For this review, take the finished solid that the model builds, in its own axes (mm). Face numbers are marked on the shaded views. A direction names the side the tool comes from. Coordinates: 2 decimals unless noted, no trailing zeros. Write each loop counter-clockwise with the first axis right and the second up, starting at its lowest first coordinate (ties: lowest second). Pieces come first, ordered by that corner, then holes. Notation, with made-up numbers: M 49.25,17.25 L 54.25,17.25 A25 cw 54.25,33.25 Z; hole C 53,-0.75 d9. An arc over 180 degrees is marked long. One line per question, with ' | ' between items.
Autodesk Inventor part; units mm, degrees
ref_plane "YZ Plane" through (0, 0, 0) normal (1, 0, 0) x (0, 1, 0)
ref_plane "XZ Plane" through (0, 0, 0) normal (0, 1, 0) x (-1, 0, 0)
ref_plane "XY Plane" through (0, 0, 0) normal (0, 0, 1) x (1, 0, 0)
sketch "Sketch1" plane through (0, 0, 0) normal (0, 0, 1) x (1, 0, 0)
  line L0 (-33.6, 0) -> (33.6, 0) construction
  line L1 (0, -33.6) -> (0, 33.6) construction
  circle A0 centre (0, 0) radius 24
  dimension "d0" = 48
extrude "Выдавливание1" add sketch "Sketch1" along normal blind 10
hole "Отверстие1" at (0, 0, 10) direction (0, 0, -1) diameter 28.376 end through all
sketch "Sketch2" plane through (0, 0, 10) normal (0, 0, 1) x (1, 0, 0)
  circle A0 centre (0, 0) radius 24
  circle A1 centre (0, 0) radius 19 construction
  line L0 (-33.6, 0) -> (33.6, 0) construction
  line L1 (0, -33.6) -> (0, 33.6) construction
  point P0 (-19, 0)
  point P1 (0, 19)
  point P2 (19, 0)
  point P3 (0, -19)
  dimension "d13" = 38
hole "Отверстие2" at (-19, 0, 10) at (0, 19, 10) at (19, 0, 10) at (0, -19, 10) direction (0, 0, -1) diameter 4.5 depth 7 tip angle 118
chamfer "Фаска1" distance 0.6 angle 45 4 edges at (0, -16.75, 10) (-19, 2.25, 10) (19, 2.25, 10) (0, 21.25, 10)
chamfer "Фаска2" distance 1 angle 45 2 edges at (-24, 0, 10) (-24, 0, 0)
sketch "Sketch3" plane through (0, 0, 0) normal (1, 0, 0) x (0, 1, 0)
  line L0 (-14.188, 0) -> (-14.188, 10) construction
  line L1 (14.188, 0) -> (14.188, 10) construction
  line L2 (-15, 10) -> (0, -5)
  line L3 (-15, 10) -> (0, 10)
  line L4 (0, 10) -> (0, -5)
  line L5 (0, -9) -> (0, 19) construction
  line L6 (-15.6074, 5) -> (15.0846, 5) construction
  line L7 (-21.7458, 0) -> (21.223, 0) construction
  line L8 (-15, 0) -> (0, 15)
  line L9 (-15, 0) -> (0, 0)
  line L10 (0, 0) -> (0, 15)
  point P0 (14.188, 5)
  dimension "d30" = 10
  dimension "d31" = 30
  dimension "d32" = 45
  dimension "d34" = 5
revolve "Вращение1" cut sketch "Sketch3" angle 360 about axis through (0, 0, -10) along (0, 0, 1)
equation "\"d0\" = D_L"
equation "\"d2\" = m_"
equation "\"d13\" = D_x"
equation "\"d14\" = d1"
equation "\"d16\" = d1"
equation "\"d19\" = h_"
equation "\"d21\" = c1"
equation "\"d24\" = c_"
equation "\"d30\" = m_"
equation "\"d31\" = d_"
equation "\"d34\" = 0.5 * m_"
equation "\"d_\" = 30"
equation "\"D_L\" = 48"
equation "\"D_x\" = 38"
equation "\"d1\" = 4.5"
equation "\"m_\" = 10"
equation "\"h_\" = 7"
equation "\"c_\" = 1"
equation "\"c1\" = 0.6"
properties part number "Гайка M30x1.5 6H ГОСТ 6393-73" material "Сталь, мягкая"
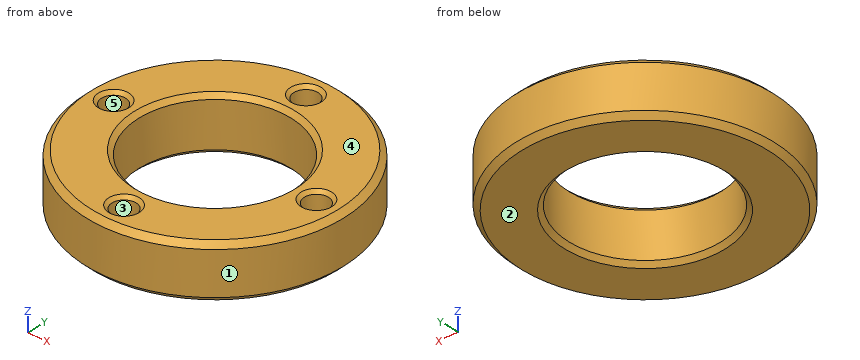
1) Machinability: for the marked faces 4 and 5, which of the approach directions +Z, -Z, +X, -X, +Y, -Y give a long, thin tool a straight path to every point of the face, cutting with its end or side? Answer none if there is none.
Responses:
face 4: +Z, +X, -X, +Y, -Y | face 5: +Z
2) Insertion check: pin 1 Ø4 at (x, y) = (0, -19) entering from -Z; pin 2 Ø3.5 at (x, y) = (0, 19) entering from +Z; pin 3 Ø5 at (x, z) = (-7.5, 8) entering from +Y; pin 4 Ø17 at (x, y) = (0, 0) entering from -Z. Each pin has a flat end and moves straight along its axis. Give the tip position at first contact, or say it passes through.
Responses:
pin 1: z = 0 | pin 2: z = 2.7 | pin 3: y = 23.47 | pin 4: through
3) We need section A-A on z = 4.75. State the section outline as (x, y) points.
Responses:
outline: C 0,0 d48; hole C -19,0 d4.5; hole C 0,0 d28.38; hole C 0,-19 d4.5; hole C 0,19 d4.5; hole C 19,0 d4.5
4) To check wall thickness, follow line 1 along X through (y, z) = (-2, 8.5); line 2 along X through (y, z) = (1.5, 7.25); line 3 along Y through (x, z) = (-19, 5.5). State the ranges of each line that lie inside material, in increasing order. Write a range as [from, to].
Responses:
line 1: [-23.92, -20.03], [-17.97, -14.05], [14.05, 17.97], [20.03, 23.92] | line 2: [-23.95, -20.68], [-17.32, -14.11], [14.11, 17.32], [20.68, 23.95] | line 3: [-14.66, -2.25], [2.25, 14.66]
5) The part is to be moulded in two halves that separate along Y. For the marked faces 1, 2 and 3, say which applies: +Y half, -Y half, draft (parallel to the pull), parting line (faces both ways), or undercut.
Responses:
face 1: parting line | face 2: draft | face 3: undercut
